Can you work these out from the model? Positions are in its coordinate system, mm. Coordinates: 2 decimals unless noted, no trailing zeros. Write each loop counter-clockwise with the first axis right and the second up, starting at its lowest first coordinate (ties: lowest second). Pieces come first, ordered by that corner, then holes.
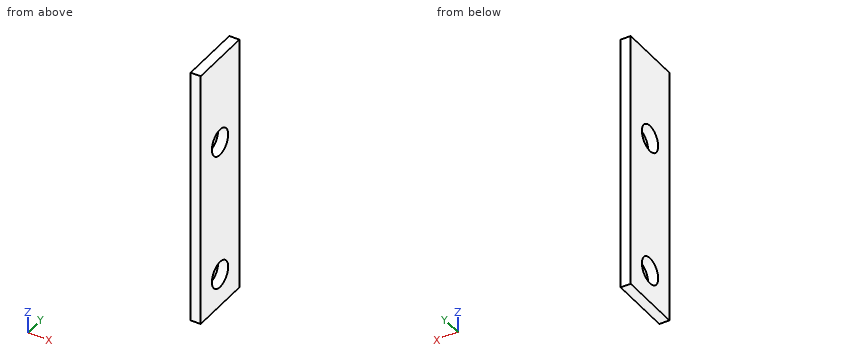
```python
from build123d import *

# Parameters (mm, degrees)
F0_W     = 25
F0_H     = 103
F0_R     = 5.25
F1_DEPTH = 4


with BuildPart() as f1:
    # F0 (on Right) → F1 (new body)
    with BuildSketch(Plane.YZ):
        Rectangle(F0_W, F0_H)
        with Locations((0, -38.5)):
            Circle(F0_R, mode=Mode.SUBTRACT)
        with Locations((0, 16.5)):
            Circle(F0_R, mode=Mode.SUBTRACT)
    extrude(amount=F1_DEPTH)


solid = f1.part
```
1. If we section it at B-B, the plane z = -38.5: List the corners of the cut face in (x, y) for me.
2. I'm going to push a flat-ended pin straight in: P1, Ø13.5, axis at y = 0, z = -38.5, coming from the -X side. Where does the tip first touch, or does it pass through?
3. If we section it at A-A, the plane y = 0: List the corners of the cut face in (x, z) for me.
4. If I drill on L1, parallel to Z at x = 2.45, y = 0; L2, parallel to Z at x = 3.05, y = -2.5; L3, parallel to Y at x = 2.9, z = -37, over which ranges is the centre line in solid material (lowest first)?
5. If we section it at C-C, the plane x = 3.2: List the corners of the cut face in (y, z) for me, plus the area to 3 significant figures.
Answers:
1. outline: (0, -12.5) - (4, -12.5) - (4, -5.25) - (0, -5.25) - close; (0, 5.25) - (4, 5.25) - (4, 12.5) - (0, 12.5) - close
2. P1: stops at x = 0
3. outline: (0, -51.5) - (4, -51.5) - (4, -43.75) - (0, -43.75) - close; (0, -33.25) - (4, -33.25) - (4, 11.25) - (0, 11.25) - close; (0, 21.75) - (4, 21.75) - (4, 51.5) - (0, 51.5) - close
4. L1: z = -51.5 to -43.75, -33.25 to 11.25, 21.75 to 51.5
4. L2: z = -51.5 to -43.12, -33.88 to 11.88, 21.12 to 51.5
4. L3: y = -12.5 to -5.03, 5.03 to 12.5
5. outline: (-12.5, -51.5) - (12.5, -51.5) - (12.5, 51.5) - (-12.5, 51.5) - close; hole circle Ø10.5 at (0, -38.5); hole circle Ø10.5 at (0, 16.5)
5. area: 2,400 mm2
